from build123d import *

# Parameters (mm, degrees)
SKETCH1_R                     = 63.5
SKETCH1_R_2                   = 38.1
BOSS_EXTRUDE1_DEPTH           = 0.762
SKETCH2_R                     = 3.175
BOSS_EXTRUDE2_DEPTH           = 26.162
CHAMFER1_SIZE                 = 25.4
CHAMFER1_SIZE2                = 2.794
CIRPATTERN3_COUNT             = 3
CHAMFER1_OF_CIRPATTERN3_SIZE2 = 2.794
CHAMFER1_OF_CIRPATTERN3_SIZE  = 25.4


with BuildPart() as part:
    # Sketch1 → Boss-Extrude1 (new body)
    with BuildSketch(Plane.XY):
        Circle(SKETCH1_R)
        Circle(SKETCH1_R_2, mode=Mode.SUBTRACT)
    extrude(amount=BOSS_EXTRUDE1_DEPTH)

    # Sketch2 → Boss-Extrude2 (add)
    with BuildSketch(Plane.XY.offset(0.762)):
        with Locations((-53.597287335, 0)):
            Circle(SKETCH2_R)
    boss_extrude2 = extrude(amount=BOSS_EXTRUDE2_DEPTH)

    # Chamfer1
    chamfer1_edges = [part.edges().sort_by_distance(p)[0] for p in [
        (-56.772287335, 0, 26.924),
    ]]
    chamfer1_side = [part.faces().sort_by_distance(p)[0] for p in [
        (-56.772287335, 0, 13.843),
    ]]
    chamfer(chamfer1_edges, length=CHAMFER1_SIZE, length2=CHAMFER1_SIZE2, reference=chamfer1_side[0])

    # CirPattern3: Boss-Extrude2 ×3 about axis
    cirpattern3_axis = Axis((0, 0, 0), (0, 0, 1))
    for i in range(1, CIRPATTERN3_COUNT):
        add(boss_extrude2.rotate(cirpattern3_axis, i * 360 / CIRPATTERN3_COUNT))

    # Chamfer1 of CirPattern3
    chamfer1_of_cirpattern3_edges = [part.edges().sort_by_distance(p)[0] for p in [
        (28.386143667, -49.166243063, 26.924),
        (28.386143667, 49.166243063, 26.924),
    ]]
    chamfer(chamfer1_of_cirpattern3_edges, length=CHAMFER1_OF_CIRPATTERN3_SIZE, length2=CHAMFER1_OF_CIRPATTERN3_SIZE2)


solid = part.part
Verification items for the finished model (mm, model axes). A direction names the side the tool comes from. Coordinates: 2 decimals unless noted, no trailing zeros. Loops run counter-clockwise (first coordinate to the right, second up) from the corner with the lowest first, then second, coordinate; pieces in that order, holes last. Notation, with made-up numbers: (-7, 18) -> (47, 18) arc R19 cw to (47, 47) -> close; hole circle Ø6 at (32, 84). An arc over 180 degrees is marked (long way). Answer as a JSON object with one key per item and string values. Group by question number.
Item 1: Scan lines: probe 1 along Y at (x, z) = (0, 0.5); probe 2 along Z at (x, y) = (-24, -51.5); probe 3 along X at (y, z) = (2.5, 3.75). Record each from-to range of solid material in increasing order.
Item 2: Mould release check, pull along Y, two halves, no side actions. Record for faces 3 (the flat face through (27.3, -27.3, 0)), 4 (the cylindrical face through (-30.235, -23.183, 0.376)), 5 (the cylindrical face through (-56.77, 0.14, 1.14)), 6 (the cylindrical face through (28.51, -43.74, 1.14)): +Y half, -Y half, draft (parallel to the pull), parting line (faces both ways), or undercut.
Item 3: Tool access check on faces 1 (the cylindrical face through (28.26, 43.6, 1.14)), 2 (the cylindrical face through (-13.77, -61.99, 0.38)). Record the directions out of +Z, -Z, +X, -X, +Y, -Y that give a thin tool (end or side, any length) a straight path to the whole face; none if there is none.
Item 4: Sectioned sample at A-A on x = 0. Record the boundary of the cut face in (y, z), plus the area to 3 significant figures.
Item 5: Depth check by flat-ended pin: pin 1 (3 mm diameter, centred on x = -40, y = -11, fed in from +Z); pin 2 (12 mm diameter, centred on x = -18, z = 3.5, fed in from +Y); pin 3 (12 mm diameter, centred on y = 51, z = 8, fed in from -X). Enter the tip coordinate at first touch or a pass-through.
Item 6: Sectioned sample at B-B on y = 32.5. Record the boundary of the cut face in (x, z), plus the area to 3 significant figures.
Item 7: Sectioned sample at D-D on z = 18. Record the boundary of the cut face in (x, y), plus the area to 3 significant figures.
Item 8: Sectioned sample at C-C on z = 8. Record the boundary of the cut face in (x, y), plus the area to 3 significant figures.
Evaluation:
{
 "1": {"probe 1": "y = -63.5 to -38.1, 38.1 to 63.5", "probe 2": "z = 0 to 0.76", "probe 3": "x = -55.13 to -52.07"},
 "2": {"face 3": "draft", "face 4": "undercut", "face 5": "parting line", "face 6": "undercut"},
 "3": {"face 1": "+Z", "face 2": "+Z, -Z"},
 "4": {"outline": "(-63.5, 0) -> (-38.1, 0) -> (-38.1, 0.76) -> (-63.5, 0.76) -> close; (38.1, 0) -> (63.5, 0) -> (63.5, 0.76) -> (38.1, 0.76) -> close", "area": "38.7 mm²"},
 "5": {"pin 1": "stops at z = 0.76", "pin 2": "stops at y = 62.22", "pin 3": "stops at x = 23.89"},
 "6": {"outline": "(-54.55, 0) -> (-19.88, 0) -> (-19.88, 0.76) -> (-54.55, 0.76) -> close; (19.88, 0) -> (54.55, 0) -> (54.55, 0.76) -> (19.88, 0.76) -> close", "area": "52.8 mm²"},
 "7": {"outline": "circle Ø2.73 at (-53.6, 0); circle Ø2.73 at (26.8, -46.42); circle Ø2.73 at (26.8, 46.42)", "area": "17.5 mm²"},
 "8": {"outline": "circle Ø4.93 at (-53.6, 0); circle Ø4.93 at (26.8, -46.42); circle Ø4.93 at (26.8, 46.42)", "area": "57.2 mm²"}
}
